Work out the finished part from the listing and answer in its coordinate system (mm). A direction names the side the tool comes from. Coordinates: 2 decimals unless noted, no trailing zeros. Loops run counter-clockwise (first coordinate to the right, second up) from the corner with the lowest first, then second, coordinate; pieces in that order, holes last.
```python
from build123d import *

# Parameters (mm, degrees)
SKETCH_R        = 2.25
PAD_DEPTH       = 15
SKETCH001_R     = 10.6
POCKET_DEPTH    = 70.001
SKETCH002_R     = 4.6
POCKET001_DEPTH = 4
CHAMFER_SIZE    = 22


with BuildPart() as part:
    # Sketch → Pad (new body)
    with BuildSketch(Plane.XY):
        Polygon((-22.5, -35), (22.5, -35), (22.5, 5), (56.7, 5), (56.7, 25), (22.5, 25), (22.5, 35), (-22.5, 35), align=None)
        with Locations((-16.7, 30)):
            Circle(SKETCH_R, mode=Mode.SUBTRACT)
        with Locations((16.7, 30)):
            Circle(SKETCH_R, mode=Mode.SUBTRACT)
        with Locations((-16.7, -30)):
            Circle(SKETCH_R, mode=Mode.SUBTRACT)
        with Locations((16.7, -30)):
            Circle(SKETCH_R, mode=Mode.SUBTRACT)
        with Locations((-16.7, 0)):
            Circle(SKETCH_R, mode=Mode.SUBTRACT)
        with Locations((16.7, 0)):
            Circle(SKETCH_R, mode=Mode.SUBTRACT)
        with Locations((16.7, 15)):
            Circle(SKETCH_R, mode=Mode.SUBTRACT)
        with Locations((46.7, 15)):
            Circle(SKETCH_R, mode=Mode.SUBTRACT)
        with Locations((-16.7, 15)):
            Circle(SKETCH_R, mode=Mode.SUBTRACT)
        with Locations((28.3, 15)):
            Circle(SKETCH_R, mode=Mode.SUBTRACT)
    extrude(amount=PAD_DEPTH)

    # Sketch001 → Pocket (cut, through all)
    with BuildSketch(Plane.XZ.offset(35)):
        with Locations((0, 15)):
            Circle(SKETCH001_R)
    extrude(amount=-POCKET_DEPTH, mode=Mode.SUBTRACT)

    # Sketch002 → Pocket001 (cut)
    with BuildSketch(Plane.XY.offset(15)):
        with Locations((-16.7, 15)):
            Circle(SKETCH002_R)
        with Locations((16.7, 15)):
            Circle(SKETCH002_R)
        with Locations((28.3, 15)):
            Circle(SKETCH002_R)
        with Locations((46.7, 15)):
            Circle(SKETCH002_R)
    extrude(amount=-POCKET001_DEPTH, mode=Mode.SUBTRACT)

    # Chamfer
    chamfer_edges = [part.edges().sort_by_distance(p)[0] for p in [
        (22.5, 5, 7.5),
    ]]
    chamfer(chamfer_edges, length=CHAMFER_SIZE)


solid = part.part
```
1. A cutting plane is placed at D-D, the plane y = -8.5. Give the vertices of the cut face in (x, z), then the cut area to 3 significant figures.
2. A cutting plane is placed at C-C, the plane z = 3. Count the separate pieces of the cut face and the enclosed holes in it, then the cut area to 3 significant figures.
3. Determine the mould class of faces 1 (the flat face through (26, 14, 11)), 2 (the flat face through (28, 8, 15)), 3 (the flat face through (-22.5, 0, 7)) for opening direction X: released by +X, released by -X, zero draft, split by the parting line, or undercut.
4. Straight lines are drawn through the part: probe 1 along Y at (x, z) = (-16.7, 6.5); probe 2 along X at (y, z) = (15, 2.75); probe 3 along Y at (x, z) = (-16.7, 11.25). For each, find the intervals that lie inside material, in ascending order.
5. A cutting plane is placed at B-B, the plane x = -16.7. Give the vertices of the cut face in (y, z), then the cut area to 3 significant figures.
6. A cutting plane is placed at A-A, the plane y = -30. Give the vertices of the cut face in (x, z).
7. Each of these flat-tipped pins is pushed along its axis until it touches: P1, Ø5, axis at x = -16.7, y = 30, coming from the +Z side; P2, Ø7.5, axis at x = 16.7, y = 15, coming from the +Z side; P3, Ø8, axis at y = -15.5, z = 2, coming from the +X side; P4, Ø4.5, axis at y = -26.5, z = 5, coming from the +X side. Where does it stop, or does it pass through?
8. For faces 4 (the flat face through (22.5, -26, 7)), 5 (the cylindrical face through (51.09, 16.38, 13.03)), 6 (the flat face through (0, 35, 4)), 7 (the flat face through (40, 25, 7)), determine the directions among +Z, -Z, +X, -X, +Y, -Y from which every point of the face is accessible in a straight line to the end or side of a thin tool.
Answers below:
1. outline: (-22.5, 0) - (31, 0) - (31, 15) - (10.6, 15) arc R10.6 cw to (-10.6, 15) - (-22.5, 15) - close
1. area: 626 mm2
2. separate pieces: 1
2. enclosed holes: 10
2. area: 3,920 mm2
3. face 1: undercut
3. face 2: zero draft
3. face 3: released by -X
4. probe 1: y = -35 to -32.25, -27.75 to -2.25, 2.25 to 12.75, 17.25 to 27.75, 32.25 to 35
4. probe 2: x = -22.5 to -18.95, -14.45 to 14.45, 18.95 to 26.05, 30.55 to 44.45, 48.95 to 56.7
4. probe 3: y = -35 to -32.25, -27.75 to -2.25, 2.25 to 10.4, 19.6 to 27.75, 32.25 to 35
5. outline: (-35, 0) - (-32.25, 0) - (-32.25, 15) - (-35, 15) - close; (-27.75, 0) - (-2.25, 0) - (-2.25, 15) - (-27.75, 15) - close; (2.25, 0) - (12.75, 0) - (12.75, 11) - (10.4, 11) - (10.4, 15) - (2.25, 15) - close; (17.25, 0) - (27.75, 0) - (27.75, 15) - (19.6, 15) - (19.6, 11) - (17.25, 11) - close; (32.25, 0) - (35, 0) - (35, 15) - (32.25, 15) - close
5. area: 761 mm2
6. outline: (-22.5, 0) - (-18.95, 0) - (-18.95, 15) - (-22.5, 15) - close; (-14.45, 0) - (14.45, 0) - (14.45, 15) - (10.6, 15) arc R10.6 cw to (-10.6, 15) - (-14.45, 15) - close; (18.95, 0) - (22.5, 0) - (22.5, 15) - (18.95, 15) - close
7. P1: stops at z = 15
7. P2: stops at z = 11
7. P3: stops at x = 28
7. P4: stops at x = 22.5
8. face 4: +Z, -Z, +X, -Y
8. face 5: +Z
8. face 6: +Z, -Z, +X, -X, +Y
8. face 7: +Z, -Z, +X, +Y
